```python
from build123d import *

# Parameters (mm, degrees)
BOSS_EXTRUDE6_DEPTH = 40
CUT_EXTRUDE2_DEPTH  = 34.5


with BuildPart() as part:
    # Sketch1 → Boss-Extrude6 (new body)
    with BuildSketch(Plane(origin=(0, 0, 0), x_dir=(1, 0, 0), z_dir=(0, 1, 0))):
        with BuildLine():
            Line((-35.196356555, 67.823627432), (-70.196356555, 67.823627432))
            Line((-70.196356555, 67.823627432), (-70.196356555, 40.323627432))
            ThreePointArc((-70.196356555, 40.323627432), (-73.125288743, 33.25255962), (-80.196356555, 30.323627432))
            Line((-80.196356555, 30.323627432), (-107.696356555, 30.323627432))
            Line((-107.696356555, 30.323627432), (-107.696356555, -4.676372568))
            Line((-107.696356555, -4.676372568), (-80.196356555, -4.676372568))
            ThreePointArc((-80.196356555, -4.676372568), (-73.125288743, -7.605304756), (-70.196356555, -14.676372568))
            Line((-70.196356555, -14.676372568), (-70.196356555, -42.176372568))
            Line((-70.196356555, -42.176372568), (-35.196356555, -42.176372568))
            Line((-35.196356555, -42.176372568), (-35.196356555, -14.676372568))
            ThreePointArc((-35.196356555, -14.676372568), (-32.267424367, -7.605304756), (-25.196356555, -4.676372568))
            Line((-25.196356555, -4.676372568), (2.303643445, -4.676372568))
            Line((2.303643445, -4.676372568), (2.303643445, 30.323627432))
            Line((2.303643445, 30.323627432), (-25.196356555, 30.323627432))
            ThreePointArc((-25.196356555, 30.323627432), (-32.267424367, 33.25255962), (-35.196356555, 40.323627432))
            Line((-35.196356555, 40.323627432), (-35.196356555, 67.823627432))
        make_face()
        Polygon((-35.196356555, -4.676372568), (-35.194570886, -4.676372568), (-35.196356555, -4.678158237), align=None, mode=Mode.SUBTRACT)
    extrude(amount=BOSS_EXTRUDE6_DEPTH)

    # Sketch1_9 → Cut-Extrude2 (cut)
    with BuildSketch(Plane(origin=(0, 0, 0), x_dir=(1, 0, 0), z_dir=(0, 1, 0))):
        with BuildLine():
            Line((-35.196356555, 65.325413101), (-70.196356555, 30.325413101))
            Line((-70.196356555, 30.325413101), (-105.198142224, -4.676372568))
            Line((-105.198142224, -4.676372568), (-80.196356555, -4.676372568))
            ThreePointArc((-80.196356555, -4.676372568), (-73.125288743, -7.605304756), (-70.196356555, -14.676372568))
            Line((-70.196356555, -14.676372568), (-70.196356555, -39.678158237))
            Line((-70.196356555, -39.678158237), (-35.196356555, -4.678158237))
            Line((-35.196356555, -4.678158237), (-35.196356555, -4.676372568))
            Line((-35.196356555, -4.676372568), (-35.194570886, -4.676372568))
            Line((-35.194570886, -4.676372568), (-0.194570886, 30.323627432))
            Line((-0.194570886, 30.323627432), (-25.196356555, 30.323627432))
            ThreePointArc((-25.196356555, 30.323627432), (-32.267424367, 33.25255962), (-35.196356555, 40.323627432))
            Line((-35.196356555, 40.323627432), (-35.196356555, 65.325413101))
        make_face()
    extrude(amount=CUT_EXTRUDE2_DEPTH, mode=Mode.SUBTRACT)


solid = part.part
```
Model file for the job. Use its own axes, mm. A direction names the side the tool comes from. Give positions to 0.01 mm unless a question says otherwise; leave off trailing zeros. Loops run counter-clockwise (first coordinate to the right, second up) from the corner with the lowest first, then second, coordinate; pieces in that order, holes last. Notation, with made-up numbers: M -22.75,-36 L 24.25,-36 A13 cw 24.25,-17 Z; hole C -14,-17.5 d10. An arc over 180 degrees is marked long. Use one line per item in the form item = value.
Item 1: Flat gauge pins, fed straight in: pin 1 Ø12 at (x, z) = (-70.5, 1.5) entering from -Y; pin 2 Ø8 at (x, y) = (-15.5, 17) entering from -Z; pin 3 Ø13.5 at (y, z) = (26, -53) entering from -X. Where does each tip first touch, or does it go through?
Filled in:
pin_1 = 34.5
pin_2 = -19.02
pin_3 = -70.2
Item 2: Which spindle directions (+Z, -Z, +X, -X, +Y, -Y) get a long thin tool onto all of the face, cutting with end or side? Do faces 1 (the flat face through (-99, 35, 4.676)), 2 (the flat face through (-12, 20, 4.676)), 3 (the flat face through (-35.196, 35, -57)), 4 (the flat face through (-53, 34.5, -9)). Say none if no direction does.
Filled in:
face_1 = +Z, -X, +Y, -Y
face_2 = +Z, +X, +Y, -Y
face_3 = -Z, +X, +Y, -Y
face_4 = -Y
Item 3: Slice it at D-D on x = -28. List the corners of the cut face in (y, z).
Filled in:
outline = M 0,-2.52 L 34.5,-2.52 L 34.5,-30.72 L 40,-30.72 L 40,5.08 L 0,5.08 Z
Item 4: Two-plate mould, pull along Z, no slides. Class faces 5 (the cylindrical face through (-73.05, 19.72, -33.33)), 6 (the flat face through (-69.71, 17.01, -30.81)), 7 (the flat face through (-70.196, 35, 31)): released by +Z, released by -Z, zero draft, split by the parting line, or undercut.
Filled in:
face_5 = released by -Z
face_6 = undercut
face_7 = zero draft
Item 5: Drill centre lines: L1, parallel to Y at x = -58.5, z = 16; L2, parallel to Z at x = -46, y = 25.5; L3, parallel to X at y = 34, z = -15. Where is each one in solid material? Low to high.
Filled in:
L1 = 34.5 to 40
L2 = -67.82 to -54.52, 15.48 to 42.18
L3 = -107.7 to -85.52, -15.52 to 2.3
Item 6: Slice it at C-C on z = 1. List the corners of the cut face in (x, y), and give its area (3 significant figures).
Filled in:
outline = M -107.7,0 L -101.52,0 L -101.52,34.5 L -31.52,34.5 L -31.52,0 L 2.3,0 L 2.3,40 L -107.7,40 Z
area = 1,980 mm^2
Item 7: Slice it at A-A on y = 33. List the corners of the cut face in (x, z), and give its area (3 significant figures).
Filled in:
outline = M -107.7,-30.32 L -80.2,-30.32 A10 cw -70.2,-40.32 L -70.2,-67.82 L -35.2,-67.82 L -35.2,-65.33 L -105.2,4.68 L -107.7,4.68 Z; M -70.2,39.68 L -0.19,-30.32 L 2.3,-30.32 L 2.3,4.68 L -25.2,4.68 A10 cw -35.2,14.68 L -35.2,42.18 L -70.2,42.18 Z
area = 2,840 mm^2
Item 8: Slice it at B-B on x = -43. List the corners of the cut face in (y, z).
Filled in:
outline = M 0,-67.82 L 40,-67.82 L 40,42.18 L 0,42.18 L 0,12.48 L 34.5,12.48 L 34.5,-57.52 L 0,-57.52 Z
